Check sheet for the modelled part. Datum: model origin and axes. Units: mm. A direction names the side the tool comes from. Give positions to 0.01 mm unless a question says otherwise; leave off trailing zeros. Write each loop counter-clockwise with the first axis right and the second up, starting at its lowest first coordinate (ties: lowest second). Pieces come first, ordered by that corner, then holes.
from build123d import *

# Parameters (mm, degrees)
BOSS_EXTRUDE1_DEPTH                     = 18
CUT_EXTRUDE1_REACH                      = 263.628
SKETCH3_W                               = 45
SKETCH3_H                               = 12
FILLET1_R                               = 25
FILLET2_R                               = 10
SKETCH4_R                               = 20
CUT_EXTRUDE2_DEPTH                      = 12
CUT_EXTRUDE3_REACH                      = 265.479
SKETCH5_R                               = 13
CHAMFER1_SIZE                           = 2
CBORE_FOR_M5_HEX_HEAD_BOLT1_D           = 5.5
CBORE_FOR_M5_HEX_HEAD_BOLT1_CBORE_D     = 12.24
CBORE_FOR_M5_HEX_HEAD_BOLT1_CBORE_DEPTH = 3.58
F_3_0MM_DOWEL_HOLE1_D                   = 3
F_3_0MM_DOWEL_HOLE1_DEPTH               = 20
F_3_0MM_DOWEL_HOLE1_TIP                 = 0.901290929


with BuildPart() as part:
    # Sketch1 → Boss-Extrude1 (new, symmetric)
    with BuildSketch(Plane.XY):
        Polygon((0, 0), (-30, 0), (-30, 185), (-90, 185), (-90, 245), (0, 245), align=None)
    extrude(amount=BOSS_EXTRUDE1_DEPTH, both=True)

    # Sketch3 → Cut-Extrude1 (cut, up to next)
    with BuildSketch(Plane(origin=(0, 245, 0), x_dir=(1, 0, 0), z_dir=(0, 1, 0)), mode=Mode.PRIVATE) as cut_extrude1_sk1:
        with Locations((-67.5, 0)):
            Rectangle(SKETCH3_W, SKETCH3_H)
    cut_extrude1_tool1 = extrude(cut_extrude1_sk1.sketch, amount=-CUT_EXTRUDE1_REACH, mode=Mode.PRIVATE) & part.part
    add(cut_extrude1_tool1.solids().sort_by_distance((-67.5, 245, 0))[0], mode=Mode.SUBTRACT)

    # Fillet1
    fillet1_edges = [part.edges().sort_by_distance(p)[0] for p in [
        (0, 245, 0),
    ]]
    fillet(fillet1_edges, radius=FILLET1_R)

    # Fillet2
    fillet2_edges = [part.edges().sort_by_distance(p)[0] for p in [
        (-30, 185, 0),
    ]]
    fillet(fillet2_edges, radius=FILLET2_R)

    # Sketch4 → Cut-Extrude2 (cut)
    with BuildSketch(Plane.XY.offset(18)):
        with Locations((-60, 215)):
            Circle(SKETCH4_R)
    extrude(amount=-CUT_EXTRUDE2_DEPTH, mode=Mode.SUBTRACT)

    # Sketch5 → Cut-Extrude3 (cut, up to next)
    with BuildSketch(Plane(origin=(0, 0, -18), x_dir=(-1, 0, 0), z_dir=(0, 0, -1)), mode=Mode.PRIVATE) as cut_extrude3_sk1:
        with Locations((60, 215)):
            Circle(SKETCH5_R)
    cut_extrude3_tool1 = extrude(cut_extrude3_sk1.sketch, amount=-CUT_EXTRUDE3_REACH, mode=Mode.PRIVATE) & part.part
    add(cut_extrude3_tool1.solids().sort_by_distance((-60, 215, -18))[0], mode=Mode.SUBTRACT)

    # Chamfer1
    chamfer1_edges = [part.edges().sort_by_distance(p)[0] for p in [
        (-65, 185, -18),
        (-57.5, 245, 18),
        (-7.32233047, 237.67766953, 18),
        (-57.5, 245, -18),
        (-7.32233047, 237.67766953, -18),
        (-30, 87.5, 18),
        (-30, 87.5, -18),
        (-32.928932188, 182.071067812, 18),
        (-32.928932188, 182.071067812, -18),
        (0, 110, -18),
        (-65, 185, 18),
        (0, 110, 18),
    ]]
    chamfer(chamfer1_edges, length=CHAMFER1_SIZE)

    # CBORE for M5 Hex Head Bolt1 (through all)
    with Locations(Plane(origin=(0, 0, 0), x_dir=(0, 0, -1), z_dir=(1, 0, 0))):
        with Locations((0, 10)):
            CounterBoreHole(CBORE_FOR_M5_HEX_HEAD_BOLT1_D / 2, CBORE_FOR_M5_HEX_HEAD_BOLT1_CBORE_D / 2, CBORE_FOR_M5_HEX_HEAD_BOLT1_CBORE_DEPTH)

    # Ø3.0mm Dowel Hole1
    with Locations(Plane.ZY.offset(90)):
        with Locations((12, 240), (-12, 190), (-12, 240), (12, 190)):
            Hole(F_3_0MM_DOWEL_HOLE1_D / 2, depth=F_3_0MM_DOWEL_HOLE1_DEPTH)
            with Locations((0, 0, -(F_3_0MM_DOWEL_HOLE1_DEPTH + F_3_0MM_DOWEL_HOLE1_TIP / 2))):  # 118° drill point
                Cone(0, F_3_0MM_DOWEL_HOLE1_D / 2, F_3_0MM_DOWEL_HOLE1_TIP, mode=Mode.SUBTRACT)


solid = part.part
1) Sectioned sample at C-C on y = 10. Record the boundary of the cut face in (x, z).
2) Sectioned sample at B-B on z = 0. Record the boundary of the cut face in (x, y).
3) Scan lines: L1, parallel to Y at x = -82.5, z = -12; L2, parallel to X at y = 216, z = 16; L3, parallel to Y at x = -81, z = 11. Record each from-to range of solid material in increasing order.
4) Gauge pin test, flat ends, axial feed: pin 1 (5.5 mm diameter, centred on x = -43.5, y = 216, fed in from +Z); pin 2 (5 mm diameter, centred on y = 240, z = 12, fed in from +X); pin 3 (3.5 mm diameter, centred on y = 240, z = -12, fed in from +X). Record the tip position at first contact, or that the pin passes through.
5) Sectioned sample at D-D on y = 124.5. Record the boundary of the cut face in (x, z), then the cut area to 3 significant figures.
6) Access from +Z, -Z, +X, -X, +Y, -Y to the whole of each face (thin tool, end or side, straight path). Record for faces 1 (the conical face through (-8.69, 236.67, 17.68)), 2 (the flat face through (-73, 222, -6)), 3 (the cylindrical face through (-62.6, 234.83, 12.08)).
7) Sectioned sample at A-A on x = -60. Record the boundary of the cut face in (y, z), then the cut area to 3 significant figures.
8) Draft check along Y on faces 4 (the flat face through (-30, 86, 0)), 5 (the cylindrical face through (-33.01, 182.15, -0.22)), 6 (the flat face through (-3.58, 9, -3)). Enter one of: +Y half, -Y half, draft (parallel to the pull), parting line (faces both ways), or undercut.
Answers below:
1. outline: (-30, -16) - (-28, -18) - (-2, -18) - (0, -16) - (0, -6.12) - (-3.58, -6.12) - (-3.58, -2.75) - (-30, -2.75) - close; (-30, 2.75) - (-3.58, 2.75) - (-3.58, 6.12) - (0, 6.12) - (0, 16) - (-2, 18) - (-28, 18) - (-30, 16) - close
2. outline: (-45, 185) - (-40, 185) arc R10 cw to (-30, 175) - (-30, 12.75) - (-3.58, 12.75) - (-3.58, 16.12) - (0, 16.12) - (0, 220) arc R25 ccw to (-25, 245) - (-45, 245) - close; (-30, 0) - (0, 0) - (0, 3.88) - (-3.58, 3.88) - (-3.58, 7.25) - (-30, 7.25) - close
3. L1: y = 185 to 188.5, 191.5 to 238.5, 241.5 to 245
3. L2: x = -90 to -79.97, -40.03 to 0
3. L3: y = 185 to 188.88, 191.12 to 238.88, 241.12 to 245
4. pin 1: stops at z = 6
4. pin 2: stops at x = -7.15
4. pin 3: stops at x = -7.91
5. outline: (-30, -16) - (-28, -18) - (-2, -18) - (0, -16) - (0, 16) - (-2, 18) - (-28, 18) - (-30, 16) - close
5. area: 1,070 mm2
6. face 1: +Z, +X, +Y
6. face 2: -X, +Y, -Y
6. face 3: +Z
7. outline: (185, -16) - (187, -18) - (202, -18) - (202, -6) - (185, -6) - close; (185, 6) - (195, 6) - (195, 18) - (187, 18) - (185, 16) - close; (228, -18) - (243, -18) - (245, -16) - (245, -6) - (228, -6) - close; (235, 6) - (245, 6) - (245, 16) - (243, 18) - (235, 18) - close
7. area: 640 mm2
8. face 4: draft
8. face 5: -Y half
8. face 6: undercut
